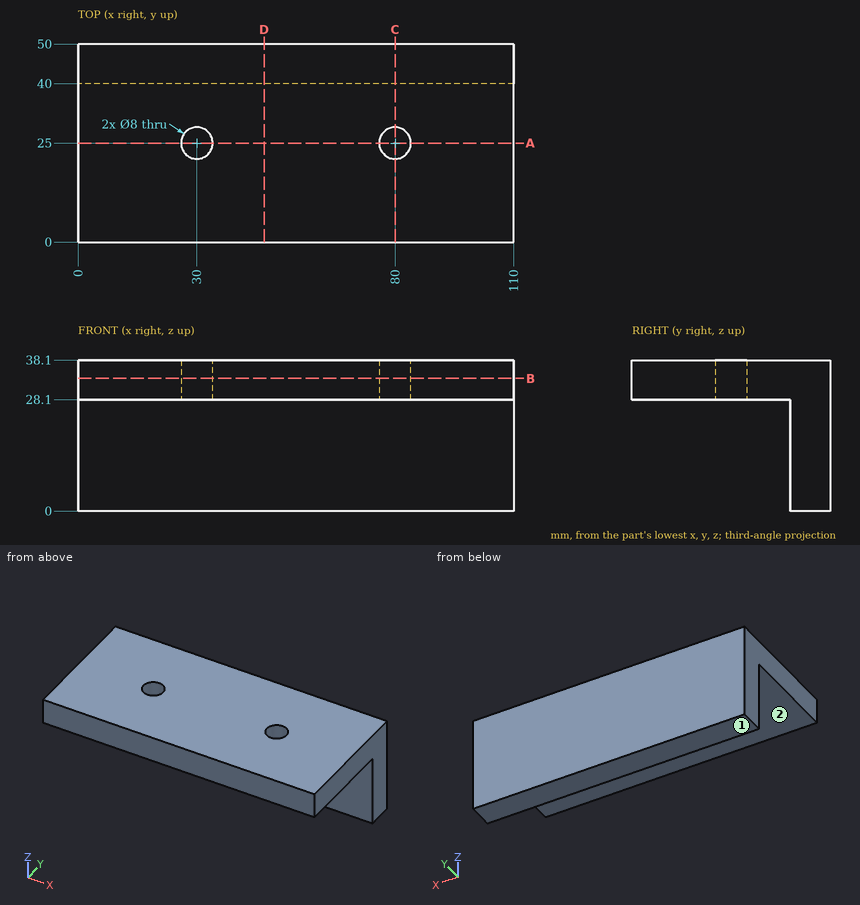
Job drawing, mm, ordinate dimensions from the low corner. One solid piece. A direction names the side the tool comes from. Round coordinates to 2 decimals unless told otherwise and drop trailing zeros. Loops run counter-clockwise (first coordinate to the right, second up) from the corner with the lowest first, then second, coordinate; pieces in that order, holes last. Notation, with made-up numbers: (14.5, -24) -> (52.5, -24) arc R26 cw to (52.5, -5) -> close; hole circle Ø7 at (-7.5, 34). An arc over 180 degrees is marked (long way). Use CSV: the item, a comma, the result in double quotes. Start each with the question number.
Q1. Drill centre lines: L1, parallel to Y at x = 80, z = 33; L2, parallel to Y at x = 24, z = 5.5; L3, parallel to Z at x = 51.5, y = 30.5. Where is each one in solid material? Low to high.
Q2. Saw through at A-A on y = 25. Give the cut face in (x, z).
Q3. Saw through at D-D on x = 47. Give the cut face in (y, z), and give its area (3 significant figures).
Q4. Saw through at C-C on x = 80. Give the cut face in (y, z), and give its area (3 significant figures).
Q5. Which spindle directions (+Z, -Z, +X, -X, +Y, -Y) get a long thin tool onto all of the face, cutting with end or side? Do the marked faces 1 and 2. Say none if no direction does.
Q6. Flat gauge pins, fed straight in: pin 1 Ø6 at (x, y) = (85.5, 7) entering from -Z; pin 2 Ø22.5 at (x, z) = (54.5, 13.5) entering from -Y. Where does each tip first touch, or does it go through?
Q7. Saw through at B-B on z = 33.5. Give the cut face in (x, y), and give its area (3 significant figures).
Solutions:
1,L1,"y = 0 to 21, 29 to 50"
1,L2,"y = 40 to 50"
1,L3,"z = 28.1 to 38.1"
2,outline,"(0, 28.1) -> (26, 28.1) -> (26, 38.1) -> (0, 38.1) -> close; (34, 28.1) -> (76, 28.1) -> (76, 38.1) -> (34, 38.1) -> close; (84, 28.1) -> (110, 28.1) -> (110, 38.1) -> (84, 38.1) -> close"
3,outline,"(0, 28.1) -> (40, 28.1) -> (40, 0) -> (50, 0) -> (50, 38.1) -> (0, 38.1) -> close"
3,area,"781 mm^2"
4,outline,"(0, 28.1) -> (21, 28.1) -> (21, 38.1) -> (0, 38.1) -> close; (29, 28.1) -> (40, 28.1) -> (40, 0) -> (50, 0) -> (50, 38.1) -> (29, 38.1) -> close"
4,area,"701 mm^2"
5,face 1,"-Z, +X, -X, +Y, -Y"
5,face 2,"-Z, +X, -X, -Y"
6,pin 1,"stops at z = 28.1"
6,pin 2,"stops at y = 40"
7,outline,"(0, 0) -> (110, 0) -> (110, 50) -> (0, 50) -> close; hole circle Ø8 at (30, 25); hole circle Ø8 at (80, 25)"
7,area,"5,400 mm^2"
